from build123d import *

# Parameters (mm, degrees)
F0_W     = 60
F0_H     = 10
F1_DEPTH = 40
F2_W     = 60
F2_H     = 20
F3_DEPTH = 10
F4_W     = 40
F4_H     = 20
F5_DEPTH = 20
F6_R     = 19.99999
F7_R     = 10
F8_R     = 10
F9_DEPTH = 25


# Not quite as in the source:
# - a fillet or chamfer is up to 0.001 mm smaller than in the source, because OpenCascade refuses the exact size


with BuildPart() as f1:
    # F0 (on Front) → F1 (new body)
    with BuildSketch(Plane.XZ):
        with Locations((30, 5)):
            Rectangle(F0_W, F0_H)
    extrude(amount=F1_DEPTH)

    # F2 (on face) → F3 (join)
    with BuildSketch(Plane.XY.offset(10)):
        with Locations((30, -10)):
            Rectangle(F2_W, F2_H)
    extrude(amount=F3_DEPTH)

    # F4 (on face) → F5 (join)
    with BuildSketch(Plane.XY.offset(20)):
        with Locations((20, -10)):
            Rectangle(F4_W, F4_H)
    extrude(amount=F5_DEPTH)

    # F6 (radius 20 in the source; OpenCascade refuses exactly that, so slightly less here)
    f6_edges = [f1.edges().sort_by_distance(p)[0] for p in [
        (0, -10, 40),
        (40, -10, 40),
    ]]
    fillet(f6_edges, radius=F6_R)

    # F7
    f7_edges = [f1.edges().sort_by_distance(p)[0] for p in [
        (60, -10, 20),
    ]]
    fillet(f7_edges, radius=F7_R)

    # F8 (on face) → F9 (cut)
    with BuildSketch(Plane.XZ.offset(20)):
        with Locations((20, 20)):
            Circle(F8_R)
    extrude(amount=-F9_DEPTH, mode=Mode.SUBTRACT)


solid = f1.part
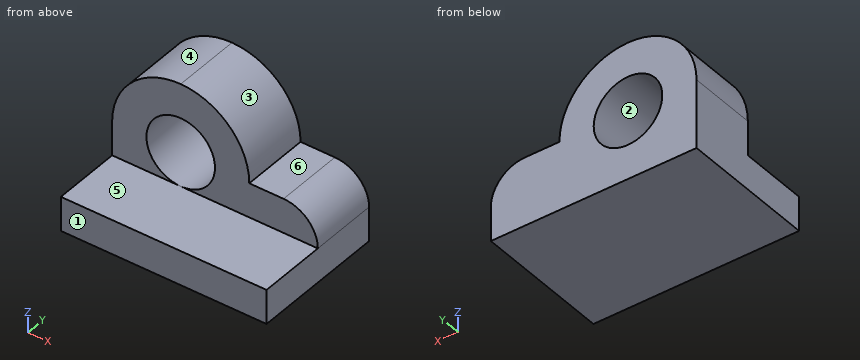
Input: part model. Units: mm. Frame: model coordinates. Face numbers are marked on the shaded views. A direction names the side the tool comes from. Round coordinates to 2 decimals unless told otherwise and drop trailing zeros. Write each loop counter-clockwise with the first axis right and the second up, starting at its lowest first coordinate (ties: lowest second). Pieces come first, ordered by that corner, then holes.
1) Reachability of the marked faces 4, 5 and 6 from +Z, -Z, +X, -X, +Y, -Y: full face, straight path, thin tool, end or side. Return the list, or none.
2) Draft query along X for the marked faces 1, 2 and 3. Return one class per face: pulls with the +X half, pulls with the -X half, needs draft (parallel to the pull), parting line crosses it, or undercut.
3) Cut plane C-C (x = 11.5). Return the cut outline in (y, z).
4) Cut plane D-D (x = 47.5). Return the cut outline in (y, z), then the cut area to 3 significant figures.
5) Cut plane B-B (z = 28). Return the cut outline in (x, y).
6) Ray query, L1, parallel to Z at x = 20, y = -13.5; L2, parallel to Y at x = 36.5, z = 17; L3, parallel to Z at x = 9.5, y = -24. Return the intervals inside material, ascending.
7) Contact query for flat-ended pins moving along their axis: P1, Ø12, axis at y = -31.5, z = 21, coming from the -X side; P2, Ø6, axis at x = 33, y = -25.5, coming from the +Z side; P3, Ø15, axis at x = 19.5, z = 31, coming from the -Y side. Output: stop coordinate, or through.
Geometry says:
1. face 4: +Z, -X, +Y, -Y
1. face 5: +Z, +X, -X, -Y
1. face 6: +Z, +X, +Y, -Y
2. face 1: needs draft
2. face 2: undercut
2. face 3: pulls with the +X half
3. outline: (-40, 0) - (0, 0) - (0, 14.73) - (-20, 14.73) - (-20, 10) - (-40, 10) - close; (-20, 25.27) - (0, 25.27) - (0, 38.1) - (-20, 38.1) - close
4. outline: (-40, 0) - (0, 0) - (0, 20) - (-20, 20) - (-20, 10) - (-40, 10) - close
4. area: 600 mm2
5. outline: (1.67, -20) - (14, -20) - (14, 0) - (1.67, 0) - close; (26, -20) - (38.33, -20) - (38.33, 0) - (26, 0) - close
6. L1: z = 0 to 10, 30 to 40
6. L2: y = -20 to 0
6. L3: z = 0 to 10
7. P1: passes through
7. P2: stops at z = 10
7. P3: stops at y = -20
